Check sheet for the modelled part. Datum: model origin and axes. Units: mm. Face numbers are marked on the shaded views. A direction names the side the tool comes from. Give positions to 0.01 mm unless a question says otherwise; leave off trailing zeros. Write each loop counter-clockwise with the first axis right and the second up, starting at its lowest first coordinate (ties: lowest second). Pieces come first, ordered by that corner, then holes.
from build123d import *

# Parameters (mm, degrees)
SKETCH1_R           = 5
SKETCH1_R_2         = 2.25
BOSS_EXTRUDE1_DEPTH = 3
BOSS_EXTRUDE2_START = 10
SKETCH2_R           = 5
SKETCH2_R_2         = 3
BOSS_EXTRUDE2_DEPTH = 10
SKETCH3_R           = 6
SKETCH3_R_2         = 4
BOSS_EXTRUDE3_DEPTH = 30
FILLET1_R           = 10
BOSS_EXTRUDE4_START = -5
SKETCH4_R           = 4
SKETCH4_R_2         = 1
BOSS_EXTRUDE4_DEPTH = 5


with BuildPart() as part:
    # Sketch1 → Boss-Extrude1 (new body)
    with BuildSketch(Plane(origin=(0, 0, 0), x_dir=(1, 0, 0), z_dir=(0, 1, 0))):
        with Locations(Location((0, 0, 0), (0, 0, 270))):
            Circle(SKETCH1_R)
        with Locations(Location((0, 0, 0), (0, 0, 270))):
            Circle(SKETCH1_R_2, mode=Mode.SUBTRACT)
    extrude(amount=BOSS_EXTRUDE1_DEPTH)

    # Sketch2 → Boss-Extrude2 (add)
    with BuildSketch(Plane.XZ.offset(BOSS_EXTRUDE2_START)):
        with Locations(Location((0, 0, 0), (0, 0, 270))):
            Circle(SKETCH2_R)
        with Locations(Location((0, 0, 0), (0, 0, 270))):
            Circle(SKETCH2_R_2, mode=Mode.SUBTRACT)
    extrude(amount=-BOSS_EXTRUDE2_DEPTH)

    # Sketch3 → Boss-Extrude3 (add)
    with BuildSketch(Plane(origin=(0, 3, 0), x_dir=(1, 0, 0), z_dir=(0, 1, 0))):
        with Locations(Location((0, 0, 0), (0, 0, 270))):
            Circle(SKETCH3_R)
        with Locations(Location((0, 0, 0), (0, 0, 270))):
            Circle(SKETCH3_R_2, mode=Mode.SUBTRACT)
    extrude(amount=BOSS_EXTRUDE3_DEPTH)

    # Fillet1
    # the kernel refuses this fillet: 10 mm, written as the material it adds along each edge
    with BuildSketch(Plane(origin=(0, 3, 0), x_dir=(0, 0, 1), z_dir=(-1, 0, 0))) as fillet1_piece_1:
        with BuildLine():
            CenterArc((15, -4.358898944), FILLET1_R, 154.158067237, 25.841932763)
            Line((6, 0), (5.82, 0.087177979))
            ThreePointArc((5.82, 0.087177979), (5.5, 0.2), (5, 0.2))
            Line((5, 0.2), (4.8, 0))
            Line((4.8, 0), (4.8, -4.358898944))
            Line((4.8, -4.358898944), (5, -4.358898944))
        make_face()
    revolve(axis=Axis((0, 3, 0), (0, 1, 0)))

    # Sketch4 → Boss-Extrude4 (add)
    with BuildSketch(Plane(origin=(0, 33, 0), x_dir=(1, 0, 0), z_dir=(0, 1, 0)).offset(BOSS_EXTRUDE4_START)):
        with BuildLine():
            Line((-8, 0), (-8, 7))
            ThreePointArc((-8, 7), (-7.707106781, 7.707106781), (-7, 8))
            Line((-7, 8), (7, 8))
            ThreePointArc((7, 8), (7.707106781, 7.707106781), (8, 7))
            Line((8, 7), (8, -7))
            ThreePointArc((8, -7), (7.707106781, -7.707106781), (7, -8))
            Line((7, -8), (-7, -8))
            ThreePointArc((-7, -8), (-7.707106781, -7.707106781), (-8, -7))
            Line((-8, -7), (-8, 0))
        make_face()
        with Locations(Location((0, 0, 0), (0, 0, 270))):
            Circle(SKETCH4_R, mode=Mode.SUBTRACT)
        with Locations(Location((-5, 5, 0), (0, 0, 270))):
            Circle(SKETCH4_R_2, mode=Mode.SUBTRACT)
        with Locations(Location((5, 5, 0), (0, 0, 270))):
            Circle(SKETCH4_R_2, mode=Mode.SUBTRACT)
        with Locations(Location((-5, -5, 0), (0, 0, 270))):
            Circle(SKETCH4_R_2, mode=Mode.SUBTRACT)
        with Locations(Location((5, -5, 0), (0, 0, 270))):
            Circle(SKETCH4_R_2, mode=Mode.SUBTRACT)
    extrude(amount=BOSS_EXTRUDE4_DEPTH)


solid = part.part
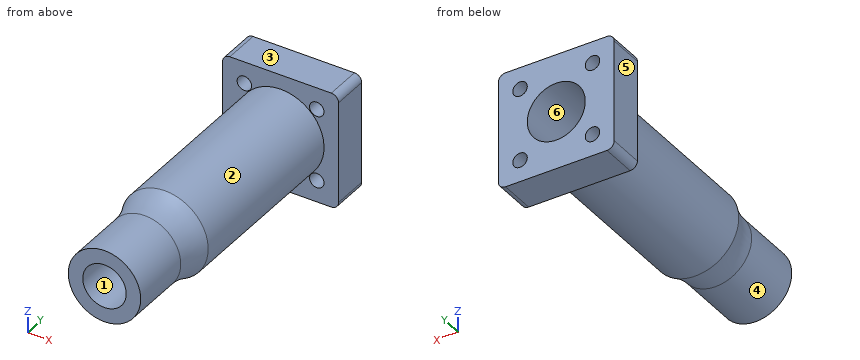
1) Sectioned sample at B-B on y = 10.5. Record the boundary of the cut face in (x, z).
2) Gauge pin test, flat ends, axial feed: pin 1 (1 mm diameter, centred on x = -0.5, y = 19.5, fed in from -Z); pin 2 (4 mm diameter, centred on x = -1, z = -1, fed in from +Y); pin 3 (7 mm diameter, centred on x = 0, z = 0, fed in from -Y); pin 4 (1.8 mm diameter, centred on x = 5, z = -5, fed in from -Y). Record the tip position at first contact, or that the pin passes through.
3) Draft check along X on the marked faces 1, 2 and 3. Enter one of: +X half, -X half, draft (parallel to the pull), parting line (faces both ways), or undercut.
4) Access from +Z, -Z, +X, -X, +Y, -Y to the whole of each face (thin tool, end or side, straight path). Record for the marked faces 4, 5 and 6.
5) Scan lines: L1, parallel to X at y = -6, z = 0; L2, parallel to Y at x = -6.5, z = 3.25; L3, parallel to X at y = -3.5, z = 1.75. Record each from-to range of solid material in increasing order.
6) Sectioned sample at A-A on x = 0. Record the boundary of the cut face in (y, z), then the cut area to 3 significant figures.
Answers below:
1. outline: circle Ø12 at (0, 0); hole circle Ø8 at (0, 0)
2. pin 1: stops at z = -6
2. pin 2: stops at y = 3
2. pin 3: stops at y = -10
2. pin 4: passes through
3. face 1: undercut
3. face 2: parting line
3. face 3: draft
4. face 4: -Y
4. face 5: +Z, -Z, -X, +Y, -Y
4. face 6: +Y
5. L1: x = -5 to -3, 3 to 5
5. L2: y = 28 to 33
5. L3: x = -4.68 to -2.44, 2.44 to 4.68
6. outline: (-10, -5) - (-1.36, -5) arc R10 cw to (3, -6) - (28, -6) - (28, -8) - (33, -8) - (33, -4) - (3, -4) - (3, -2.25) - (0, -2.25) - (0, -3) - (-10, -3) - close; (-10, 3) - (0, 3) - (0, 2.25) - (3, 2.25) - (3, 4) - (33, 4) - (33, 8) - (28, 8) - (28, 6) - (3, 6) arc R10 cw to (-1.36, 5) - (-10, 5) - close
6. area: 199 mm2
